from build123d import *

# Parameters (mm, degrees)
SKETCH1_W           = 50.8
SKETCH1_H           = 25.4
SKETCH1_W_2         = 44.45
SKETCH1_H_2         = 19.05
BOSS_EXTRUDE1_DEPTH = 66.04
SKETCH2_R           = 2.0193
SKETCH2_R_2         = 6.35
CUT_EXTRUDE1_DEPTH  = 63.5
SKETCH3_R           = 2.0193
CUT_EXTRUDE2_DEPTH  = 63.5


with BuildPart() as part:
    # Sketch1 → Boss-Extrude1 (new body)
    with BuildSketch(Plane.XY):
        with Locations((25.4, 12.7)):
            Rectangle(SKETCH1_W, SKETCH1_H)
        with Locations((25.4, 12.7)):
            Rectangle(SKETCH1_W_2, SKETCH1_H_2, mode=Mode.SUBTRACT)
    extrude(amount=BOSS_EXTRUDE1_DEPTH)

    # Sketch2 → Cut-Extrude1 (cut)
    with BuildSketch(Plane(origin=(0, 25.4, 0), x_dir=(1, 0, 0), z_dir=(0, 1, 0))):
        with Locations((12.7, -53.34)):
            Circle(SKETCH2_R)
        with Locations((25.4, -46.99)):
            Circle(SKETCH2_R_2)
        with Locations((38.1, -53.34)):
            Circle(SKETCH2_R)
        with Locations((12.7, -40.64)):
            Circle(SKETCH2_R)
        with Locations((38.1, -40.64)):
            Circle(SKETCH2_R)
        with Locations((12.7, -27.94)):
            Circle(SKETCH2_R)
        with Locations((38.1, -27.94)):
            Circle(SKETCH2_R)
        with Locations((12.7, -15.24)):
            Circle(SKETCH2_R)
        with Locations((38.1, -15.24)):
            Circle(SKETCH2_R)
        with Locations((25.4, -21.59)):
            Circle(SKETCH2_R_2)
    extrude(amount=-CUT_EXTRUDE1_DEPTH, mode=Mode.SUBTRACT)

    # Sketch3 → Cut-Extrude2 (cut)
    with BuildSketch(Plane(origin=(50.8, 0, 0), x_dir=(0, 0, -1), z_dir=(1, 0, 0))):
        with Locations((-53.34, 12.7)):
            Circle(SKETCH3_R)
        with Locations((-40.64, 12.7)):
            Circle(SKETCH3_R)
        with Locations((-27.94, 12.7)):
            Circle(SKETCH3_R)
        with Locations((-15.24, 12.7)):
            Circle(SKETCH3_R)
    extrude(amount=-CUT_EXTRUDE2_DEPTH, mode=Mode.SUBTRACT)


solid = part.part
Geometry: final body of the model. Coordinates: model frame, mm. A direction names the side the tool comes from. Give positions to 0.01 mm unless a question says otherwise; leave off trailing zeros. Write each loop counter-clockwise with the first axis right and the second up, starting at its lowest first coordinate (ties: lowest second). Pieces come first, ordered by that corner, then holes.
(1) First-contact query: P1, Ø3, axis at y = 12.7, z = 15.24, coming from the -X side. Flat tip, straight axial feed; report the tip coordinate or a pass-through.
(2) Ray query, line 1 (Z direction, x = 25.4, y = 23.7); line 2 (Z direction, x = 38.1, y = 22.9); line 3 (Y direction, x = 12, z = 59) (3 decimals). Return the intervals inside material, ascending.
(3) Cut plane C-C, the plane x = 25.4. Return loops of the section in (y, z) (3 decimals).
(4) Cut plane B-B, the plane y = 16. Return loops of the section in (x, z) (3 decimals), then the cut area to 3 significant figures.
(5) Cut plane D-D, the plane y = 1.75. Give the number of separate pieces and of enclosed holes in the cut face, then the cut area to 3 significant figures.
(6) Access query for faces 5 (the flat face through (47.625, 13, 33)), 6 (the cylindrical face through (49.235, 12.789, 55.357)). Directions: +Z, -Z, +X, -X, +Y, -Y. A direction counts if a zero-diameter tool reaches every point of the face in a straight line with its end or side. Return the directions, or none.
(7) Cut plane A-A, the plane z = 46.99. Return loops of the section in (x, y) (3 decimals), then the cut area to 3 significant figures.
(8) Mould query, pull axis Z, two halves, no side actions, for faces 1 (the cylindrical face through (36.61, 23.83, 39.28)), 2 (the cylindrical face through (36.5, 1.61, 29.17)), 3 (the flat face through (25, 23, 66.04)), 4 (the flat face through (50.8, 13, 33)). Classes: released by +Z, released by -Z, zero draft, split by the parting line, or undercut.
Values follow:
1. P1: passes through
2. line 1: z = 0 to 15.24, 27.94 to 40.64, 53.34 to 66.04
2. line 2: z = 0 to 13.22, 17.26 to 25.92, 29.96 to 38.62, 42.66 to 51.32, 55.36 to 66.04
2. line 3: y = 0 to 3.175, 22.225 to 25.4
3. outline: (0, 0) - (3.175, 0) - (3.175, 15.24) - (0, 15.24) - close; (0, 27.94) - (3.175, 27.94) - (3.175, 40.64) - (0, 40.64) - close; (0, 53.34) - (3.175, 53.34) - (3.175, 66.04) - (0, 66.04) - close; (22.225, 0) - (25.4, 0) - (25.4, 15.24) - (22.225, 15.24) - close; (22.225, 27.94) - (25.4, 27.94) - (25.4, 40.64) - (22.225, 40.64) - close; (22.225, 53.34) - (25.4, 53.34) - (25.4, 66.04) - (22.225, 66.04) - close
4. outline: (0, 0) - (3.175, 0) - (3.175, 66.04) - (0, 66.04) - close; (47.625, 0) - (50.8, 0) - (50.8, 66.04) - (47.625, 66.04) - close
4. area: 419 mm2
5. separate pieces: 1
5. enclosed holes: 10
5. area: 3,000 mm2
6. face 5: +Z, -Z
6. face 6: +X, -X
7. outline: (0, 0) - (19.05, 0) - (19.05, 3.175) - (3.175, 3.175) - (3.175, 22.225) - (19.05, 22.225) - (19.05, 25.4) - (0, 25.4) - close; (31.75, 0) - (50.8, 0) - (50.8, 25.4) - (31.75, 25.4) - (31.75, 22.225) - (47.625, 22.225) - (47.625, 3.175) - (31.75, 3.175) - close
7. area: 363 mm2
8. face 1: undercut
8. face 2: undercut
8. face 3: released by +Z
8. face 4: zero draft
